```python
from build123d import *

# Parameters (mm, degrees)
SKETCH_1_R      = 1.7
SKETCH_1_R_2    = 1.05
SKETCH_1_W      = 22.9
SKETCH_1_H      = 22.9
EXTRUDE_1_DEPTH = 2


with BuildPart() as part:
    # 草图1 → 凸台-拉伸1 (new body)
    with BuildSketch(Plane(origin=(0, 0, 0), x_dir=(1, 0, 0), z_dir=(0, 1, 0))):
        with BuildLine():
            ThreePointArc((-23.9, -18.856654127), (-22.435533906, -22.392188032), (-18.9, -23.856654127))
            Line((-18.9, -23.856654127), (18.9, -23.856654127))
            ThreePointArc((18.9, -23.856654127), (22.435533906, -22.392188032), (23.9, -18.856654127))
            Line((23.9, -18.856654127), (23.9, -0.043345873))
            Line((23.9, -0.043345873), (23.9, 0.043345873))
            Line((23.9, 0.043345873), (23.9, 18.856654127))
            ThreePointArc((23.9, 18.856654127), (22.435533906, 22.392188032), (18.9, 23.856654127))
            Line((18.9, 23.856654127), (-18.9, 23.856654127))
            ThreePointArc((-18.9, 23.856654127), (-22.435533906, 22.392188032), (-23.9, 18.856654127))
            Line((-23.9, 18.856654127), (-23.9, 0.043345873))
            Line((-23.9, 0.043345873), (-23.9, -0.043345873))
            Line((-23.9, -0.043345873), (-23.9, -18.856654127))
        make_face()
        with Locations(Location((-19.2, -19.2, 0), (0, 0, 270))):
            Circle(SKETCH_1_R, mode=Mode.SUBTRACT)
        with Locations(Location((-16.45, -11.45, 0), (0, 0, 270))):
            Circle(SKETCH_1_R_2, mode=Mode.SUBTRACT)
        with Locations(Location((19.2, -19.2, 0), (0, 0, 270))):
            Circle(SKETCH_1_R, mode=Mode.SUBTRACT)
        Rectangle(SKETCH_1_W, SKETCH_1_H, mode=Mode.SUBTRACT)
        with Locations(Location((16.45, -11.45, 0), (0, 0, 270))):
            Circle(SKETCH_1_R_2, mode=Mode.SUBTRACT)
        with Locations(Location((-16.45, 11.45, 0), (0, 0, 270))):
            Circle(SKETCH_1_R_2, mode=Mode.SUBTRACT)
        with Locations(Location((-19.2, 19.2, 0), (0, 0, 270))):
            Circle(SKETCH_1_R, mode=Mode.SUBTRACT)
        with Locations(Location((16.45, 11.45, 0), (0, 0, 270))):
            Circle(SKETCH_1_R_2, mode=Mode.SUBTRACT)
        with Locations(Location((19.2, 19.2, 0), (0, 0, 270))):
            Circle(SKETCH_1_R, mode=Mode.SUBTRACT)
    extrude(amount=EXTRUDE_1_DEPTH)


solid = part.part
```
The model under review builds one solid part; all positions refer to its coordinate system, in mm. A direction names the side the tool comes from. Round coordinates to 2 decimals unless told otherwise and drop trailing zeros. Write each loop counter-clockwise with the first axis right and the second up, starting at its lowest first coordinate (ties: lowest second). Pieces come first, ordered by that corner, then holes. Notation, with made-up numbers: (62.25, 21) -> (84.25, 21) arc R25 cw to (84.25, 50) -> close; hole circle Ø5 at (84.5, 4.5). An arc over 180 degrees is marked (long way). Use CSV: the item, a comma, the result in double quotes.
Q1. Consider section A-A (x = 4.5). Give the boundary of the cut face in (y, z).
Checks:
outline,"(0, -23.86) -> (2, -23.86) -> (2, -11.45) -> (0, -11.45) -> close; (0, 11.45) -> (2, 11.45) -> (2, 23.86) -> (0, 23.86) -> close"
Q2. Consider section B-B (z = -6.5). Give the boundary of the cut face in (x, y), then the cut area to 3 significant figures.
Checks:
outline,"(-23.9, 0) -> (-11.45, 0) -> (-11.45, 2) -> (-23.9, 2) -> close; (11.45, 0) -> (23.9, 0) -> (23.9, 2) -> (11.45, 2) -> close"
area,"49.8 mm²"
Q3. Consider section C-C (x = 16.45). Give the boundary of the cut face in (y, z).
Checks:
outline,"(0, -23.86) -> (2, -23.86) -> (2, -12.5) -> (0, -12.5) -> close; (0, -10.4) -> (2, -10.4) -> (2, 10.4) -> (0, 10.4) -> close; (0, 12.5) -> (2, 12.5) -> (2, 23.86) -> (0, 23.86) -> close"
Q4. To check wall thickness, follow probe 1 along Z at (x, y) = (-16.5, 0.3); probe 2 along X at (y, z) = (1.25, -19.2); probe 3 along X at (y, z) = (1.3, 2.5). State the ranges of each line that lie inside material, in increasing order. Write a range as [from, to].
Checks:
probe 1,"[-23.86, -12.5], [-10.4, 10.4], [12.5, 23.86]"
probe 2,"[-23.89, -20.9], [-17.5, 17.5], [20.9, 23.89]"
probe 3,"[-23.9, -11.45], [11.45, 23.9]"
Q5. For faces 1 (the flat face through (0, 1, -11.45)), 2 (the flat face through (0, 2, 16)), list the 3-axis set-ups (+Z, -Z, +X, -X, +Y, -Y) from which the entire face can be reached by the end or side of a thin tool; tool diameter is ignored.
Checks:
face 1,"+Y, -Y"
face 2,"+Z, -Z, +X, -X, +Y"
Q6. Consider section D-D (y = 0.6). State how many separate pieces and enclosed holes the cut face has, then the cut area to 3 significant figures.
Checks:
separate pieces,"1"
enclosed holes,"9"
area,"1,680 mm²"
Q7. Mouldability with a two-part tool opening along X and no side actions: class faces 3 (the cylindrical face through (-19.13, 0.99, -20.9)), 4 (the flat face through (-23.9, 1, 0)), 5 (the cylindrical face through (-17.475, 0.986, 11.222)), 6 (the flat face through (0, 0, 16)) as released by +X, released by -X, zero draft, split by the parting line, or undercut.
Checks:
face 3,"undercut"
face 4,"released by -X"
face 5,"undercut"
face 6,"zero draft"
